For this review, use the dimensioned drawing (mm, ordinates from the lowest corner) and the shaded views. A direction names the side the tool comes from. Coordinates: 2 decimals unless noted, no trailing zeros. Loops run counter-clockwise (first coordinate to the right, second up) from the corner with the lowest first, then second, coordinate; pieces in that order, holes last. Notation, with made-up numbers: (46.5, -14.75) -> (70.5, -14.75) arc R9 ccw to (70.5, 2.25) -> close; hole circle Ø8 at (-19, -2). An arc over 180 degrees is marked (long way). Answer as a JSON object with one key per item and string values.
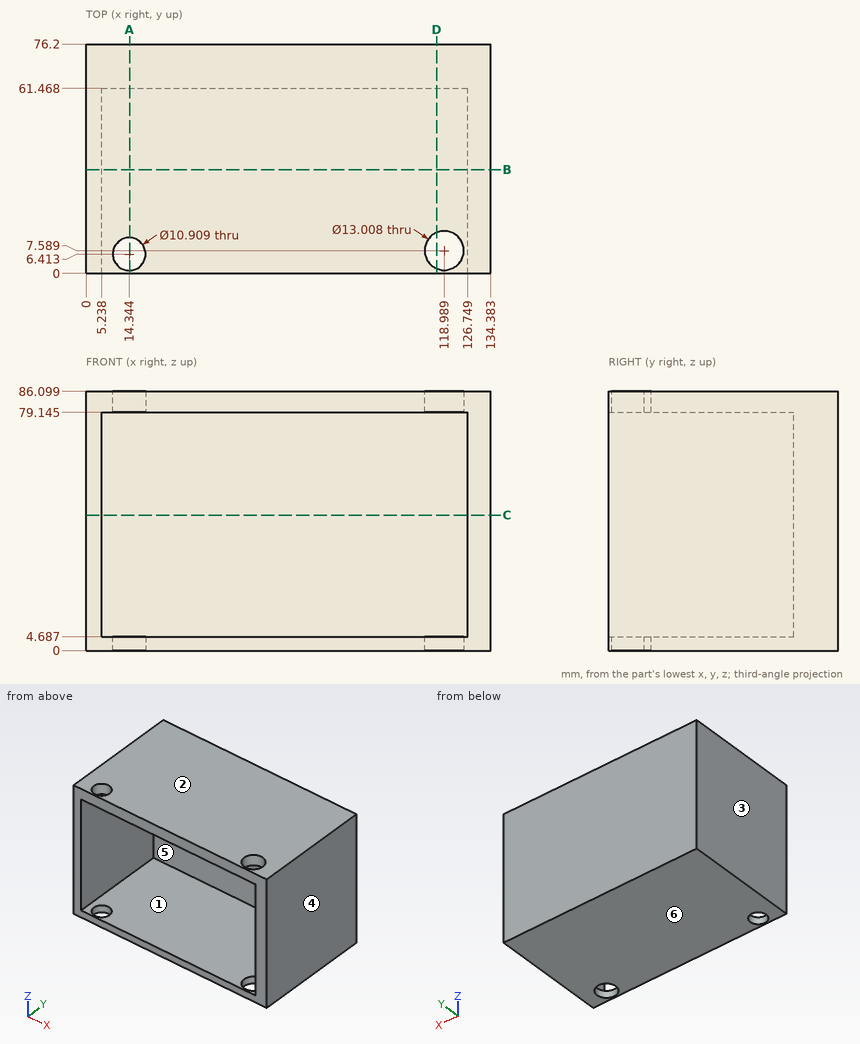
1) For the marked faces 5 and 6, list the 3-axis set-ups (+Z, -Z, +X, -X, +Y, -Y) from which the entire face can be reached by the end or side of a thin tool; tool diameter is ignored.
Completed:
{"face 5": "-Y", "face 6": "-Z, +X, -X, +Y, -Y"}
2) The part is to be moulded in two halves that separate along X. For the marked faces 1, 2, 3 and 4, say which applies: pulls with the +X half, pulls with the -X half, needs draft (parallel to the pull), parting line crosses it, or undercut.
Completed:
{"face 1": "undercut", "face 2": "needs draft", "face 3": "pulls with the -X half", "face 4": "pulls with the +X half"}
3) Clearance check with a flat-ended pin moving along its axis: pin 1 Ø4 at (x, z) = (75.5, 74.5) entering from -Y. State where the tip first meets the part, or that it passes through.
Completed:
{"pin 1": "y = 61.47"}
4) Wall thickness on probe 1 along Z at (x, y) = (83.5, 33.5) (1 decimal); probe 2 along X at (y, z) = (13, 44.5); probe 3 along Y at (x, z) = (116.5, 52): over which ranges is each line inside the solid? List them lowest first.
Completed:
{"probe 1": "0 to 4.7, 79.1 to 86.1", "probe 2": "0 to 5.24, 126.75 to 134.38", "probe 3": "61.47 to 76.2"}
5) Add section A-A, the plane x = 14.5. Give the boundary of the cut face in (y, z) (1 decimal), and give its area (3 significant figures).
Completed:
{"outline": "(0, 0) -> (1, 0) -> (1, 4.7) -> (0, 4.7) -> close; (0, 79.1) -> (1, 79.1) -> (1, 86.1) -> (0, 86.1) -> close; (11.9, 0) -> (76.2, 0) -> (76.2, 86.1) -> (11.9, 86.1) -> (11.9, 79.1) -> (61.5, 79.1) -> (61.5, 4.7) -> (11.9, 4.7) -> close", "area": "1,860 mm²"}
6) Add section B-B, the plane y = 34.5. Give the boundary of the cut face in (x, z) (1 decimal), and give its area (3 significant figures).
Completed:
{"outline": "(0, 0) -> (134.4, 0) -> (134.4, 86.1) -> (0, 86.1) -> close; hole (5.2, 4.7) -> (126.7, 4.7) -> (126.7, 79.1) -> (5.2, 79.1) -> close", "area": "2,520 mm²"}
7) Add section D-D, the plane x = 116.5. Give the boundary of the cut face in (y, z) (1 decimal).
Completed:
{"outline": "(0, 0) -> (1.6, 0) -> (1.6, 4.7) -> (0, 4.7) -> close; (0, 79.1) -> (1.6, 79.1) -> (1.6, 86.1) -> (0, 86.1) -> close; (13.6, 0) -> (76.2, 0) -> (76.2, 86.1) -> (13.6, 86.1) -> (13.6, 79.1) -> (61.5, 79.1) -> (61.5, 4.7) -> (13.6, 4.7) -> close"}
8) Add section C-C, the plane z = 45. Give the boundary of the cut face in (x, y).
Completed:
{"outline": "(0, 0) -> (5.24, 0) -> (5.24, 61.47) -> (126.75, 61.47) -> (126.75, 0) -> (134.38, 0) -> (134.38, 76.2) -> (0, 76.2) -> close"}
